from build123d import *

# Parameters (mm, degrees)
F0_R     = 25.4
F0_R_2   = 9.525
F1_DEPTH = 38.1


with BuildPart() as f1:
    # F0 (on Front) → F1 (new body)
    with BuildSketch(Plane.XZ):
        Polygon((300.096595, -135.002792), (-1338.203405, -135.002792), (-1338.203405, -185.802792), (0, -312.802792), (723.9, -312.802792), (998.643007, -262.002792), (998.643007, -109.602792), align=None)
        with Locations((-25.340905, -262.002792)):
            Circle(F0_R, mode=Mode.SUBTRACT)
        with Locations((-912.753405, -204.852792)):
            Circle(F0_R_2, mode=Mode.SUBTRACT)
    extrude(amount=F1_DEPTH)


solid = f1.part
Source: CAD feature listing. Evaluate the final solid. Frame: model axes, mm. A direction names the side the tool comes from. Coordinates: 2 decimals unless noted, no trailing zeros. Write each loop counter-clockwise with the first axis right and the second up, starting at its lowest first coordinate (ties: lowest second). Pieces come first, ordered by that corner, then holes. Notation, with made-up numbers: M 17,23 L 72,23 A22 cw 72,49 Z; hole C 1,25 d6. An arc over 180 degrees is marked long. Use a Markdown table: item, result.
1) Mould query, pull axis Z, two halves, no side actions, for faces 3 (the flat face through (654.26, -18.783, -122.125)), 4 (the cylindrical face through (-28.65, -18.78, -236.82)), 5 (the flat face through (-678.469, -18.783, -248.414)). Classes: pulls with the +Z half, pulls with the -Z half, needs draft (parallel to the pull), parting line crosses it, or undercut.
Conclusion:
| item | result |
|---|---|
| face 3 | pulls with the +Z half |
| face 4 | undercut |
| face 5 | pulls with the -Z half |
2) First-contact query: pin 1 Ø19 at (x, y) = (-846.5, -22) entering from +Z. Flat tip, straight axial feed; report the tip coordinate or a pass-through.
Conclusion:
| item | result |
|---|---|
| pin 1 | stops at z = -135 |
3) Section B-B, the plane x = 82. Output: boundary loops of the cut face in (y, z).
Conclusion:
| item | result |
|---|---|
| outline | M -38.1,-312.8 L 0,-312.8 L 0,-135 L -38.1,-135 Z |
4) Ray query, L1, parallel to Z at x = 622.5, y = -4; L2, parallel to Z at x = -859.5, y = -15. Return the intervals inside material, ascending.
Conclusion:
| item | result |
|---|---|
| L1 | z = -312.8 to -123.28 |
| L2 | z = -231.23 to -135 |
5) Section A-A, the plane y = -19.5. Output: boundary loops of the cut face in (x, z) (3 decimals), then the cut area to 3 significant figures.
Conclusion:
| item | result |
|---|---|
| outline | M -1338.203,-185.803 L 0,-312.803 L 723.9,-312.803 L 998.643,-262.003 L 998.643,-109.603 L 300.097,-135.003 L -1338.203,-135.003 Z; hole C -912.753,-204.853 d19.05; hole C -25.341,-262.003 d50.8 |
| area | 330,000 mm^2 |
6) Reachability of faces 1 (the flat face through (-508, -19, -135.003)), 2 (the flat face through (74, -38.1, -210)) from +Z, -Z, +X, -X, +Y, -Y: full face, straight path, thin tool, end or side. Return the list, or none.
Conclusion:
| item | result |
|---|---|
| face 1 | +Z, -X, +Y, -Y |
| face 2 | +Z, -Z, +X, -X, -Y |
7) Section C-C, the plane x = -326.5. Output: boundary loops of the cut face in (y, z).
Conclusion:
| item | result |
|---|---|
| outline | M -38.1,-281.82 L 0,-281.82 L 0,-135 L -38.1,-135 Z |
